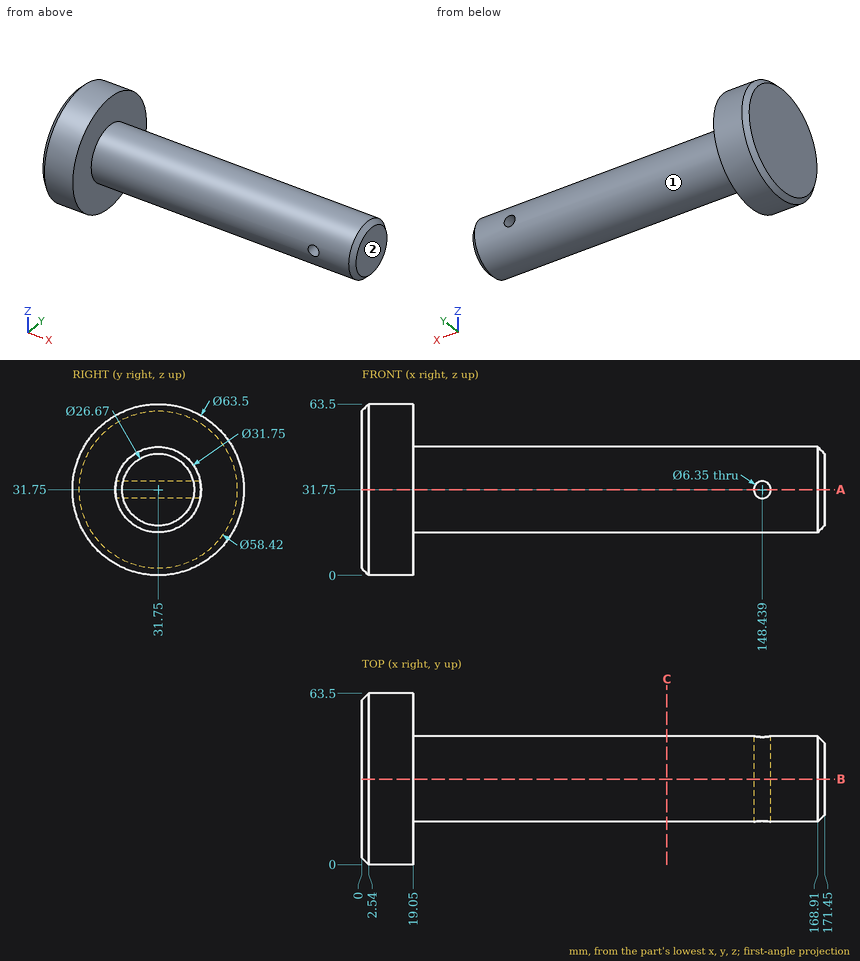
Design review of the part shown in the three views and the two pictorial views. Dimensions are in mm from the part's minimum x, y and z. A direction names the side the tool comes from. Round coordinates to 2 decimals unless told otherwise and drop trailing zeros. Loops run counter-clockwise (first coordinate to the right, second up) from the corner with the lowest first, then second, coordinate; pieces in that order, holes last.
(1) Clearance check with flat-ended pins moving along their axes: P1, Ø6, axis at y = 20.5, z = 13, coming from the +X side; P2, Ø12, axis at x = 27.5, y = 41.5, coming from the +Z side; P3, Ø1, axis at x = 138.5, y = 26.5, coming from the +Z side. State where each tip first meets the part, or that it passes through.
Returned:
P1: stops at x = 19.05
P2: stops at z = 47.18
P3: stops at z = 46.9
(2) Tool access review of the marked faces 1 and 2: name each direction out of +Z, -Z, +X, -X, +Y, -Y from which nothing blocks a thin tool from reaching the whole face with its end or side.
Returned:
face 1: +X
face 2: +Z, -Z, +X, +Y, -Y
(3) We need section B-B (y = 31.75). Give the boundary of the cut face in (x, z) (3 decimals), plus the area to 3 significant figures.
Returned:
outline: (0, 2.54) - (2.54, 0) - (19.05, 0) - (19.05, 15.875) - (168.91, 15.875) - (171.45, 18.415) - (171.45, 45.085) - (168.91, 47.625) - (19.05, 47.625) - (19.05, 63.5) - (2.54, 63.5) - (0, 60.96) - close; hole circle Ø6.35 at (148.439, 31.75)
area: 6,000 mm2
(4) Wall thickness on line 1 along X through (y, z) = (26, 31.75); line 2 along X through (y, z) = (33, 31); line 3 along X through (y, z) = (32.5, 60.5): over which ranges is each line inside the solid? List them lowest first.
Returned:
line 1: x = 0 to 145.26, 151.61 to 171.45
line 2: x = 0 to 145.35, 151.52 to 171.45
line 3: x = 0 to 19.05
(5) We need section A-A (z = 31.75). Give the boundary of the cut face in (x, y) (3 decimals), plus the area to 3 significant figures.
Returned:
outline: (0, 2.54) - (2.54, 0) - (19.05, 0) - (19.05, 15.875) - (145.264, 15.875) - (145.264, 47.625) - (19.05, 47.625) - (19.05, 63.5) - (2.54, 63.5) - (0, 60.96) - close; (151.614, 15.875) - (168.91, 15.875) - (171.45, 18.415) - (171.45, 45.085) - (168.91, 47.625) - (151.614, 47.625) - close
area: 5,830 mm2
(6) We need section C-C (x = 113). Give the boundary of the cut face in (y, z) (3 decimals), plus the area to 3 significant figures.
Returned:
outline: circle Ø31.75 at (31.75, 31.75)
area: 792 mm2
